Geometry: see drawing. Coordinates: mm, zero at the bounding-box minimum. A direction names the side the tool comes from. Round coordinates to 2 decimals unless told otherwise and drop trailing zeros. Write each loop counter-clockwise with the first axis right and the second up, starting at its lowest first coordinate (ties: lowest second). Pieces come first, ordered by that corner, then holes. Notation, with made-up numbers: M 18,33.25 L 68,33.25 A8 ccw 68,41.25 Z; hole C 86,59.25 d8. An arc over 180 degrees is marked long. Use a Markdown table: item, result.
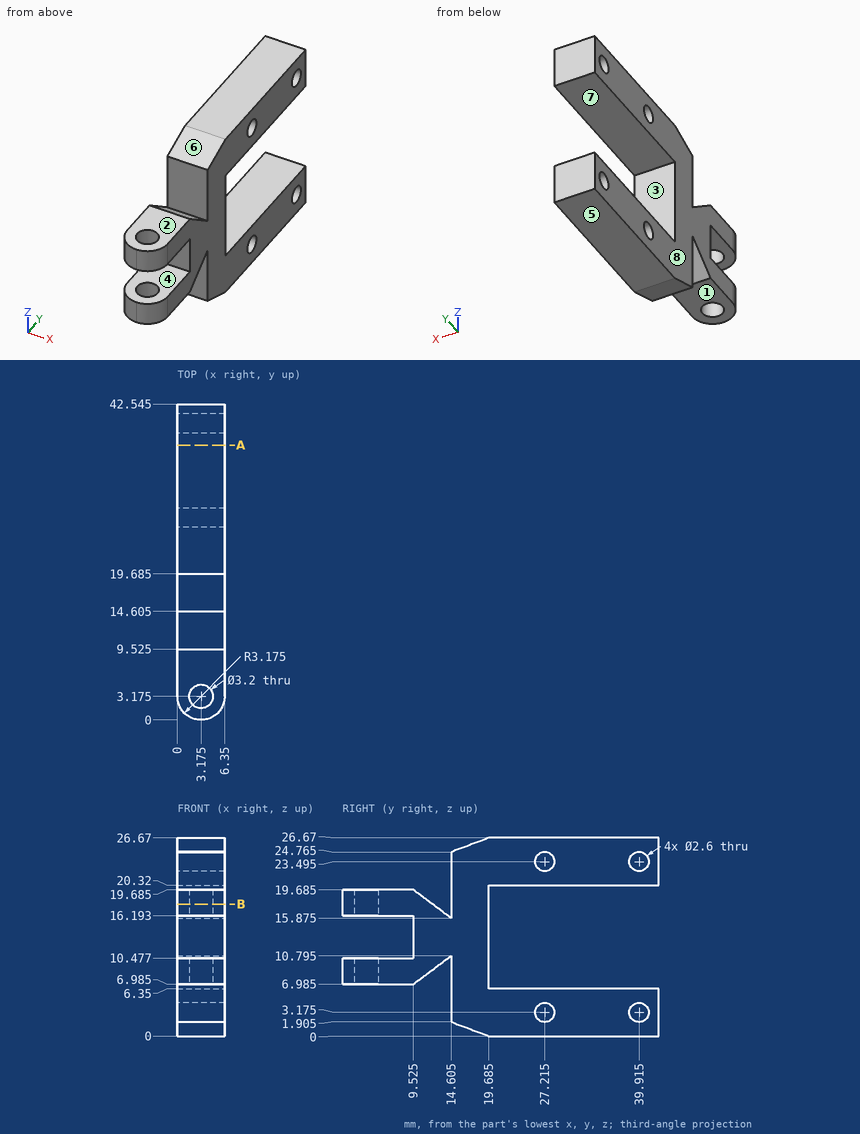
Q1. Section A-A on y = 37. Return loops of the section in (x, z).
Results are:
| item | result |
|---|---|
| outline | M 0,0 L 6.35,0 L 6.35,6.35 L 0,6.35 Z; M 0,20.32 L 6.35,20.32 L 6.35,26.67 L 0,26.67 Z |
Q2. First-contact query: pin 1 Ø1 at (x, y) = (1, 12.5) entering from +Z; pin 2 Ø3 at (x, y) = (2, 4) entering from -Z (1 decimal); pin 3 Ø1.5 at (x, z) = (4.5, 19.5) entering from -Y; pin 4 Ø2 at (y, z) = (39.91, 23.49) entering from +X (1 decimal). Flat tips, straight axial feed; report the tip coordinate or a pass-through.
Results are:
| item | result |
|---|---|
| pin 1 | z = 17.83 |
| pin 2 | z = 7 |
| pin 3 | y = 0.05 |
| pin 4 | through |
Q3. Reachability of the marked faces 1, 2, 3 and 4 from +Z, -Z, +X, -X, +Y, -Y: full face, straight path, thin tool, end or side. Return the list, or none.
Results are:
| item | result |
|---|---|
| face 1 | -Z, +X, -X, -Y |
| face 2 | +Z, +X, -X, -Y |
| face 3 | +X, -X, +Y |
| face 4 | +X, -X, -Y |
Q4. Section B-B on z = 17.75. Give the number of separate pieces and of enclosed holes in the cut face.
Results are:
| item | result |
|---|---|
| separate pieces | 2 |
| enclosed holes | 1 |
Q5. Mould query, pull axis Z, two halves, no side actions, for the marked faces 5, 6, 7 and 8. Classes: +Z half, -Z half, draft (parallel to the pull), parting line (faces both ways), or undercut.
Results are:
| item | result |
|---|---|
| face 5 | -Z half |
| face 6 | +Z half |
| face 7 | undercut |
| face 8 | draft |
Q6. Line query: L1, parallel to Y at x = 3.25, z = 17 (1 decimal); L2, parallel to Y at x = 2.75, z = 7.25 (1 decimal); L3, parallel to Z at x = 4, y = 8.5 (1 decimal). Output: solid intervals per line, ascending.
Results are:
| item | result |
|---|---|
| L1 | 0 to 1.6, 4.8 to 13.1, 14.6 to 19.7 |
| L2 | 0 to 1.6, 4.7 to 9.9, 14.6 to 19.7 |
| L3 | 7 to 10.5, 16.2 to 19.7 |
